Job drawing, mm, ordinate dimensions from the low corner. One solid piece. Give positions to 0.01 mm unless a question says otherwise; leave off trailing zeros. Order: outer loops, then holes, each group sorted by start corner. A loop starts at its lowest first (then second) coordinate and runs counter-clockwise, first axis right, second up. Notation, with made-up numbers: (14.25, -37.75) - (55.25, -37.75) arc R36 ccw to (55.25, -2.75) - close; hole circle Ø9 at (68.5, -27). An arc over 180 degrees is marked (long way). One line per item, written item: value.
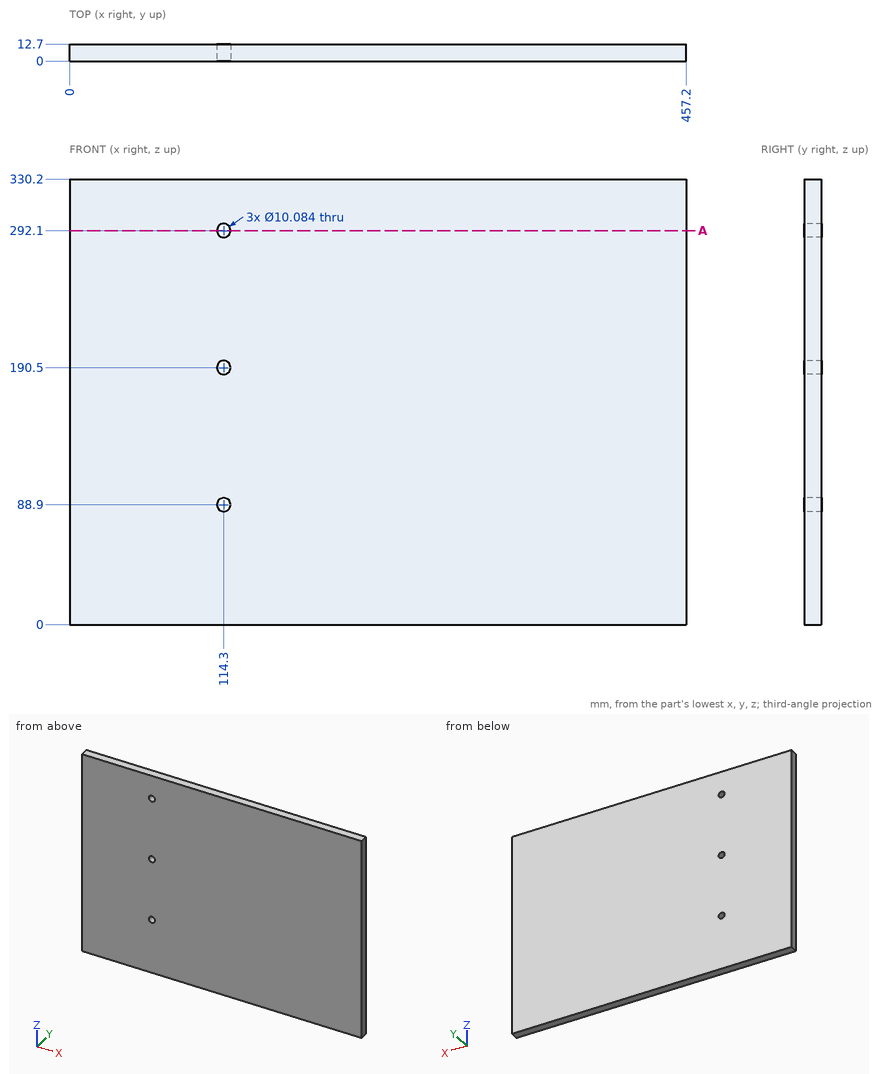
1) Slice it at A-A on z = 292.1. Write the cut outline in (x, y).
Answer:
outline: (0, 0) - (109.26, 0) - (109.26, 12.7) - (0, 12.7) - close; (119.34, 0) - (457.2, 0) - (457.2, 12.7) - (119.34, 12.7) - close
2) Wall check: line 1 along Z through (x, y) = (114.3, 9.5); line 2 along X through (y, z) = (9.5, 190.5); line 3 along X through (y, z) = (1.25, 186.5). Give the ranges that are in metal, low to high. Write a range as [from, to].
Answer:
line 1: z = [0, 83.86], [93.94, 185.46], [195.54, 287.06], [297.14, 330.2]
line 2: x = [0, 109.26], [119.34, 457.2]
line 3: x = [0, 111.23], [117.37, 457.2]
3) Drop flat-ended pins along their axis: P1, Ø5, axis at x = 366, z = 294.5, coming from the -Y side; P2, Ø6, axis at x = 114.3, z = 88.9, coming from the -Y side. Give the stop position or say it passes through.
Answer:
P1: stops at y = 0
P2: passes through
